from build123d import *
from OCP.BRepFilletAPI import BRepFilletAPI_MakeChamfer

# Parameters (mm, degrees)
SKETCH1_R           = 5.75
BOSS_EXTRUDE1_DEPTH = 3
BOSS_EXTRUDE3_DEPTH = 0.3
CIRPATTERN1_COUNT   = 2
SKETCH4_R           = 2.5
CUT_EXTRUDE1_DEPTH  = 65.609278472
CHAMFER1_SIZE       = 1
CHAMFER1_SIZE2      = 1.191753593


with BuildPart() as part:
    # Sketch1 → Boss-Extrude1 (new, symmetric)
    with BuildSketch(Plane(origin=(0, 0, 0), x_dir=(1, 0, 0), z_dir=(0, 1, 0))):
        with Locations(Location((0, 0, 0), (0, 0, 270))):
            Circle(SKETCH1_R)
    extrude(amount=BOSS_EXTRUDE1_DEPTH, both=True)

    # Sketch3 → Boss-Extrude3 (add)
    with BuildSketch(Plane(origin=(0, 0, 0), x_dir=(0.9743700647852351, -0.22495105434386534, 0), z_dir=(-0.22495105434386534, -0.9743700647852351, 0))):
        with BuildLine():
            Line((-4.869810272, -3.811414063), (-6.277481036, -7.811414063))
            Line((-6.277481036, -7.811414063), (-5.9307932, -60.519732009))
            ThreePointArc((-5.9307932, -60.519732009), (-5.045190608, -62.628285228), (-2.930858092, -63.5))
            Line((-2.930858092, -63.5), (-0.266005483, -63.5))
            ThreePointArc((-0.266005483, -63.5), (2.708645134, -62.518887124), (4.515908541, -59.960581485))
            add(Edge.make_bspline(
                [(4.515908541, -59.960581485), (16.627834102, -30.503690424), (4.515908541, -2.064662287)],
                knots=[0, 0, 0, 1, 1, 1], degree=2))
            add(Edge.make_bspline(
                [(-4.869810272, -3.811414063), (0.634471784, -8.039563779), (4.515908541, -2.064662287)],
                knots=[0, 0, 0, 1, 1, 1], degree=2))
        make_face()
    boss_extrude3 = extrude(amount=BOSS_EXTRUDE3_DEPTH)

    # CirPattern1: Boss-Extrude3 ×2 about axis
    cirpattern1_axis = Axis((0, 3, 0), (0, -1, 0))
    for i in range(1, CIRPATTERN1_COUNT):
        add(boss_extrude3.rotate(cirpattern1_axis, i * 360 / CIRPATTERN1_COUNT))

    # Sketch4 → Cut-Extrude1 (cut, through all)
    with BuildSketch(Plane(origin=(0, 3, 0), x_dir=(1, 0, 0), z_dir=(0, 1, 0))):
        with Locations(Location((0, 0, 0), (0, 0, 270))):
            Circle(SKETCH4_R)
    extrude(amount=-CUT_EXTRUDE1_DEPTH, mode=Mode.SUBTRACT)

    # Chamfer1: one chamfer whose edges measure the first distance from different faces: ONE call of the kernel's chamfer builder (chamfer() names one face for all edges)
    chamfer1_edges_1 = [part.edges().sort_by_distance(p)[0] for p in [
        (0, -3, -2.5),
    ]]
    chamfer1_side_1 = [part.faces().sort_by_distance(p)[0] for p in [
        (0, 0, -2.5),
    ]]
    chamfer1_edges_2 = [part.edges().sort_by_distance(p)[0] for p in [
        (0, 3, -2.5),
    ]]
    chamfer1_side_2 = [part.faces().sort_by_distance(p)[0] for p in [
        (0, 3, -5.58736544),
    ]]
    chamfer1 = BRepFilletAPI_MakeChamfer(part.part.solid().wrapped)
    for e in chamfer1_edges_1:
        chamfer1.Add(CHAMFER1_SIZE, CHAMFER1_SIZE2, e.wrapped, chamfer1_side_1[0].wrapped)  # the first distance lies on this face
    for e in chamfer1_edges_2:
        chamfer1.Add(CHAMFER1_SIZE, CHAMFER1_SIZE2, e.wrapped, chamfer1_side_2[0].wrapped)  # the first distance lies on this face
    add(Compound.cast(chamfer1.Shape()), mode=Mode.REPLACE)


solid = part.part
Geometry check sheet. Reference: the model listing, model coordinates, mm. A direction names the side the tool comes from. Round coordinates to 2 decimals unless told otherwise and drop trailing zeros. Order: outer loops, then holes, each group sorted by start corner. A loop starts at its lowest first (then second) coordinate and runs counter-clockwise, first axis right, second up. Notation, with made-up numbers: M 6.5,43 L 10.5,43 A22 cw 10.5,78 Z; hole C 67.5,-32 d6. An arc over 180 degrees is marked long. Answer in a Markdown table with one row per item.
(1) Scan lines: probe 1 along X at (y, z) = (-0.5, 0); probe 2 along Z at (x, y) = (-3.75, -0.75); probe 3 along Z at (x, y) = (-0.5, -0.5). Record each from-to range of solid material in increasing order. Write a range as from..to.
Responses:
| item | result |
|---|---|
| probe 1 | x = -5.75..-2.5, 2.5..5.75 |
| probe 2 | z = -4.36..4.36 |
| probe 3 | z = -5.73..-2.45, 2.45..5.73 |
(2) Go/stop test with flat-tipped pins: P1, Ø6, axis at x = -7, z = 23, coming from the -Y side; P2, Ø4, axis at x = 6, z = 20.5, coming from the -Y side; P3, Ø3, axis at x = 0, z = 0, coming from the -Y side; P4, Ø3, axis at x = 0.5, y = 0.5, coming from the +Z side. Record where each tip stops, or that it passes through.
Responses:
| item | result |
|---|---|
| P1 | stops at y = -2.59 |
| P2 | stops at y = 0.62 |
| P3 | passes through |
| P4 | stops at z = 63.5 |
(3) Sectioned sample at A-A, the plane z = 0. Record the cut outline in (x, y), and give its area (3 significant figures).
Responses:
| item | result |
|---|---|
| outline | M -5.75,-3 L -3.69,-3 L -2.5,-2 L -2.5,1.81 L -3.5,3 L -5.75,3 Z; M 2.5,-2 L 3.69,-3 L 5.75,-3 L 5.75,3 L 3.5,3 L 2.5,1.81 Z |
| area | 36.6 mm² |
(4) Draft check along X on faces 3 (the face through (0, 3, 4)), 4 (the face through (-2.44, -0.07, -0.54)). Enter one of: released by +X, released by -X, zero draft, split by the parting line, or undercut.
Responses:
| item | result |
|---|---|
| face 3 | zero draft |
| face 4 | undercut |
(5) Tool access check on faces 1 (the face through (-4, -3, 0)), 2 (the face through (3.886, 0.042, -4.238)). Record the directions out of +Z, -Z, +X, -X, +Y, -Y that give a thin tool (end or side, any length) a straight path to the whole face; none if there is none.
Responses:
| item | result |
|---|---|
| face 1 | +Z, -Z, +X, -X, -Y |
| face 2 | none |
